Read the model definition and answer for the solid it produces. Units are mm, in the model's axes. A direction names the side the tool comes from. Coordinates: 2 decimals unless noted, no trailing zeros. Write each loop counter-clockwise with the first axis right and the second up, starting at its lowest first coordinate (ties: lowest second). Pieces come first, ordered by that corner, then holes.
Item 1: A tool of negligible diameter and unlimited length cuts with its end or side. For faces 4 (the face through (0, 17.5, 394)), 5 (the face through (0, 14.5, 394)), from which of +Z, -Z, +X, -X, +Y, -Y can it reach the whole face along a straight path? Write none if from no direction.
Item 2: Section B-B (z = 200) is taken. Give the vertices of the cut face in (x, y).
Item 3: Straight lines are drawn through the part: probe 1 along Y at (x, z) = (11, 280); probe 2 along X at (y, z) = (-13.5, 363.5). For each, find the intervals that lie inside material, in ascending order.
Item 4: This flat-tipped pin is pushed along its axis until it touches: P1, Ø1, axis at y = 13, z = 537, coming from the +X side. Where does it stop, or does it pass through?
Item 5: Section A-A (x = 0.5) is taken. Give the vertices of the cut face in (y, z), then the cut area to 3 significant figures.
Item 6: Determine the mould class of faces 1 (the face through (0, -14.5, 394)), 2 (the face through (-17.5, 0, 394)), 3 (the face through (15, 0, 0)) for opening direction X: released by +X, released by -X, zero draft, split by the parting line, or undercut.
Autodesk Inventor part; units mm, degrees
ref_plane "Počáteční rovina" through (0, 0, 0) normal (0, 0, 1) x (1, 0, 0)
ref_plane "Koncová rovina" through (0, 0, 805) normal (0, 0, 1) x (1, 0, 0)
ref_plane "YZ Plane" through (0, 0, 0) normal (1, 0, 0) x (0, 1, 0)
ref_plane "Počáteční rovina" through (0, 0, 0) normal (0, 0, 1) x (1, 0, 0)
ref_plane "Koncová rovina" through (0, 0, 805) normal (0, 0, 1) x (1, 0, 0)
sketch "Náčrt1" plane through (0, 0, 0) normal (0, 0, 1) x (1, 0, 0)
  line L0 (-11.5, 17.5) -> (11.5, 17.5)
  line L1 (17.5, 11.5) -> (17.5, -11.5)
  line L2 (11.5, -17.5) -> (-11.5, -17.5)
  line L3 (-17.5, -11.5) -> (-17.5, 11.5)
  arc A0 (-11.5, 17.5) -> (-17.5, 11.5) centre (-11.5, 11.5) ccw
  arc A1 (17.5, 11.5) -> (11.5, 17.5) centre (11.5, 11.5) ccw
  arc A2 (11.5, -17.5) -> (17.5, -11.5) centre (11.5, -11.5) ccw
  arc A3 (-17.5, -11.5) -> (-11.5, -17.5) centre (-11.5, -11.5) ccw
  line L4 (-26.2397, 0) -> (26.2397, 0) construction
  line L5 (0, -26.2397) -> (0, 26.2397) construction
  arc A4 (-11.5, 14.5) -> (-14.5, 11.5) centre (-11.5, 11.5) ccw
  line L6 (-11.5, 14.5) -> (11.5, 14.5)
  arc A5 (14.5, 11.5) -> (11.5, 14.5) centre (11.5, 11.5) ccw
  line L7 (14.5, 11.5) -> (14.5, -11.5)
  arc A6 (11.5, -14.5) -> (14.5, -11.5) centre (11.5, -11.5) ccw
  line L8 (11.5, -14.5) -> (-11.5, -14.5)
  arc A7 (-14.5, -11.5) -> (-11.5, -14.5) centre (-11.5, -11.5) ccw
  line L9 (-14.5, -11.5) -> (-14.5, 11.5)
  point P0 (-17.5, 17.5)
  point P1 (17.5, -17.5)
  point P2 (17.5, 17.5)
  dimension "b" = 35
  dimension "msp_r" = 6
  dimension "d8" = 17.5
  dimension "d9" = 17.5
  dimension "d10" = 3
extrude "Těleso" add sketch "Náčrt1" along normal blind 800
sketch "Sketch2" plane through (0, 0, 0) normal (0, 0, 1) x (1, 0, 0)
  line L0 (0, 0) -> (10, 0)
ref_plane "Work Plane3" through (0, 0, 0) normal (0, -1, 0) x (1, 0, 0)
sketch "Sketch3" plane through (0, 0, 0) normal (0, -1, 0) x (1, 0, 0)
  line L0 (-2, 0) -> (12, 0)
  line L1 (-2, 805) -> (12, 805)
  dimension "d14" = 805
equation "\"msp_r\" = 2 * ParT"
equation "\"d8\" = d9"
equation "\"d9\" = 0.5 * b"
equation "\"d10\" = ParT"
equation "\"G_OFFSET_START\" = 0"
equation "\"G_OFFSET_END\" = 0"
equation "\"d12\" = G_OFFSET_END + B_L"
equation "\"G_L\" = d14"
equation "\"B_L\" = 805"
properties part number "CSN 426935 - 35x35x3-805" material "Nerezová ocel"
Established:
1. face 4: +Z, -Z, +X, -X, +Y
1. face 5: +Z, -Z
2. outline: (-17.5, -11.5) arc R6 ccw to (-11.5, -17.5) - (11.5, -17.5) arc R6 ccw to (17.5, -11.5) - (17.5, 11.5) arc R6 ccw to (11.5, 17.5) - (-11.5, 17.5) arc R6 ccw to (-17.5, 11.5) - close; hole (-14.5, -11.5) arc R3 ccw to (-11.5, -14.5) - (11.5, -14.5) arc R3 ccw to (14.5, -11.5) - (14.5, 11.5) arc R3 ccw to (11.5, 14.5) - (-11.5, 14.5) arc R3 ccw to (-14.5, 11.5) - close
3. probe 1: y = -17.5 to -14.5, 14.5 to 17.5
3. probe 2: x = -17.16 to -13.74, 13.74 to 17.16
4. P1: stops at x = 17.42
5. outline: (-17.5, 0) - (-14.5, 0) - (-14.5, 800) - (-17.5, 800) - close; (14.5, 0) - (17.5, 0) - (17.5, 800) - (14.5, 800) - close
5. area: 4,800 mm2
6. face 1: undercut
6. face 2: released by -X
6. face 3: zero draft
